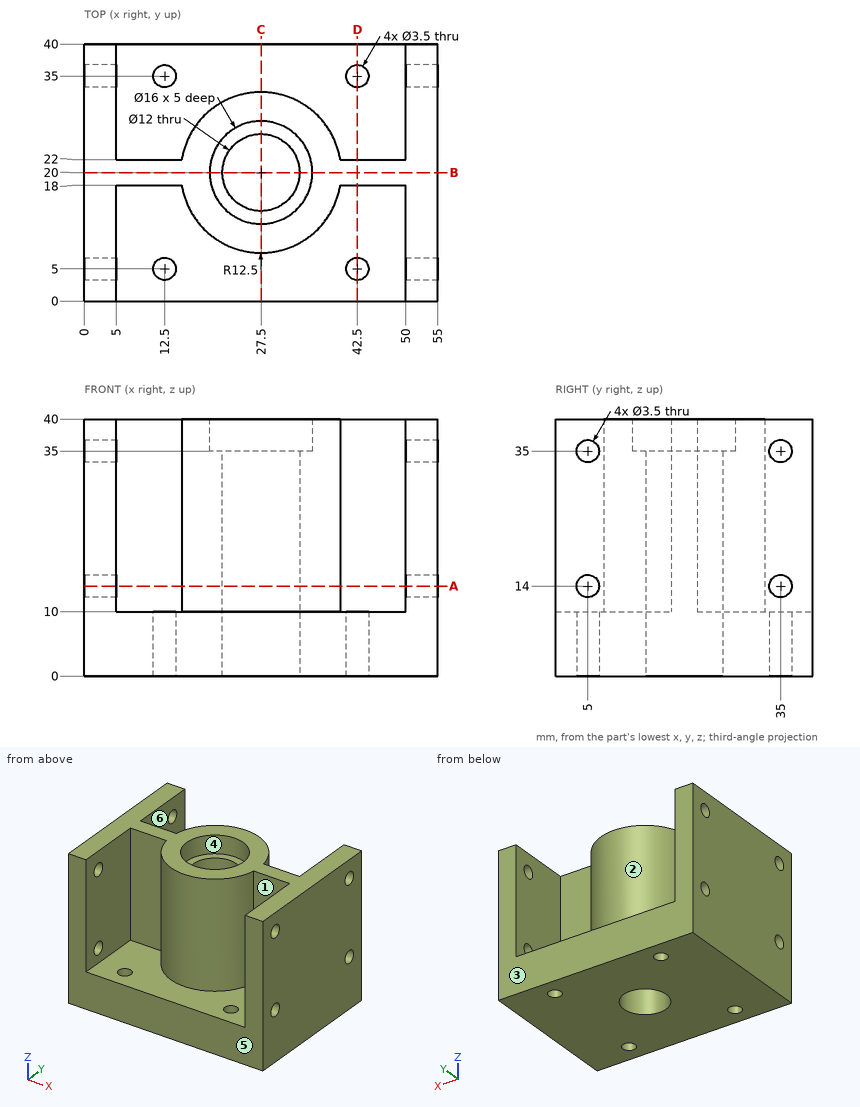
Geometry: see drawing. Coordinates: mm, zero at the bounding-box minimum. A direction names the side the tool comes from. Give positions to 0.01 mm unless a question says otherwise; leave off trailing zeros. Loops run counter-clockwise (first coordinate to the right, second up) from the corner with the lowest first, then second, coordinate; pieces in that order, holes last. Notation, with made-up numbers: (82.5, -31.75) -> (120.5, -31.75) arc R19 cw to (120.5, -16.75) -> close; hole circle Ø1 at (88.5, 25). An arc over 180 degrees is marked (long way). Put each result on its own line as item: value.
1. Cut plane C-C (x = 27.5). Return the cut outline in (y, z).
Taken from the geometry:
outline: (0, 0) -> (14, 0) -> (14, 35) -> (12, 35) -> (12, 40) -> (7.5, 40) -> (7.5, 10) -> (0, 10) -> close; (26, 0) -> (40, 0) -> (40, 10) -> (32.5, 10) -> (32.5, 40) -> (28, 40) -> (28, 35) -> (26, 35) -> close
2. Cut plane D-D (x = 42.5). Return the cut outline in (y, z).
Taken from the geometry:
outline: (0, 0) -> (3.25, 0) -> (3.25, 10) -> (0, 10) -> close; (6.75, 0) -> (33.25, 0) -> (33.25, 10) -> (22, 10) -> (22, 40) -> (18, 40) -> (18, 10) -> (6.75, 10) -> close; (36.75, 0) -> (40, 0) -> (40, 10) -> (36.75, 10) -> close
3. Cut plane B-B (y = 20). Return the cut outline in (x, z).
Taken from the geometry:
outline: (0, 0) -> (21.5, 0) -> (21.5, 35) -> (19.5, 35) -> (19.5, 40) -> (0, 40) -> close; (33.5, 0) -> (55, 0) -> (55, 40) -> (35.5, 40) -> (35.5, 35) -> (33.5, 35) -> close
4. Set-up query: the marked faces 1, 2 and 3. Return all of +Z, -Z, +X, -X, +Y, -Y with unobstructed straight access to the full face (end or side cutting, diameter ignored); none if empty.
Taken from the geometry:
face 1: +Z, -Y
face 2: +Z, +Y
face 3: +Z, -Z, +X, -X, +Y
5. Cut plane A-A (z = 14). Count the separate pieces of the cut face and the enclosed holes in it, plus the area to 3 significant figures.
Taken from the geometry:
separate pieces: 5
enclosed holes: 1
area: 788 mm2
6. Pin query (flat end, axial travel): P1, Ø3, axis at x = 39.5, z = 31.5, coming from the -Y side; P2, Ø6, axis at x = 32, z = 27, coming from the -Y side; P3, Ø8, axis at x = 10, z = 30.5, coming from the -Y side. Return the tip coordinate at first contact, or that it passes through.
Taken from the geometry:
P1: stops at y = 13.22
P2: stops at y = 7.59
P3: stops at y = 18
7. Ray query, line 1 along Z through (x, y) = (52.85, 5); line 2 along Y through (x, z) = (12.5, 3.5); line 3 along X through (y, z) = (37.5, 35). Return the intervals inside material, ascending. Write a range as [from, to].
Taken from the geometry:
line 1: z = [0, 12.25], [15.75, 33.25], [36.75, 40]
line 2: y = [0, 3.25], [6.75, 33.25], [36.75, 40]
line 3: x = [0, 5], [50, 55]
8. Pull-direction query (Y, two-part tool) for the marked faces 4, 5 and 6; classes: released by +Y, released by -Y, zero draft, split by the parting line, or undercut.
Taken from the geometry:
face 4: undercut
face 5: released by -Y
face 6: zero draft
